from build123d import *

# Parameters (mm, degrees)
SCHIZZO1_W                   = 690
SCHIZZO1_H                   = 400
ESTRUSIONE_ESTRUSIONE1_DEPTH = 10
SCHIZZO2_W                   = 690
SCHIZZO2_H                   = 400
SCHIZZO2_W_2                 = 670
SCHIZZO2_H_2                 = 380
ESTRUSIONE_ESTRUSIONE2_DEPTH = 150


with BuildPart() as part:
    # Schizzo1 → Estrusione-Estrusione1 (new body)
    with BuildSketch(Plane.XY):
        Rectangle(SCHIZZO1_W, SCHIZZO1_H)
    extrude(amount=ESTRUSIONE_ESTRUSIONE1_DEPTH)

    # Schizzo2 → Estrusione-Estrusione2 (add)
    with BuildSketch(Plane.XY.offset(10)):
        Rectangle(SCHIZZO2_W, SCHIZZO2_H)
        Rectangle(SCHIZZO2_W_2, SCHIZZO2_H_2, mode=Mode.SUBTRACT)
    extrude(amount=ESTRUSIONE_ESTRUSIONE2_DEPTH)


solid = part.part
Can you work these out from the model? Positions are in its coordinate system, mm. A direction names the side the tool comes from. Coordinates: 2 decimals unless noted, no trailing zeros. Order: outer loops, then holes, each group sorted by start corner. A loop starts at its lowest first (then second) coordinate and runs counter-clockwise, first axis right, second up. Notation, with made-up numbers: (-40, 4) - (-29, 4) arc R26 cw to (-29, 21) - close; hole circle Ø2 at (6.5, 35). An arc over 180 degrees is marked (long way). Answer as a JSON object with one key per item and string values. Group by question number.
Q1. On a 3-axis mill with a long thin cutter (end or side, diameter ignored), from which of +Z, -Z, +X, -X, +Y, -Y can I reach the whole of each face in a straight line? I mean faces 1 (the face through (-345, -3, 79)), 2 (the face through (-5, 3, 10)). Say none if no direction works.
Q2. Imagine slicing it at A-A (z = 78). Please give me the cut outline in (x, y), and give its area (3 significant figures).
Q3. We'd pull the mould along X, two halves only. Please class faces 3 (the face through (345, -3, 79)), 4 (the face through (-5, -200, 79)), 5 (the face through (335, -3, 84)): +X half, -X half, draft (parallel to the pull), parting line (faces both ways), or undercut.
Q4. I need wall thicknesses on line 1 (X direction, y = 168.5, z = 129); line 2 (Y direction, x = -67.5, z = 119); line 3 (Z direction, x = 279.5, y = -92). Which ranges of each line are inside material? Lowest first, please. Write a range as from..to.
Q5. Imagine slicing it at B-B (y = -88.5). Please give me the cut outline in (x, z), and give its area (3 significant figures).
Q6. Imagine slicing it at C-C (x = -258). Please give me the cut outline in (y, z), and give its area (3 significant figures).
Q7. Will this pin go through, and if not, where does the flat tip stop? P1, Ø12, axis at x = -160, y = -2.5, coming from the -Z side.
Determined:
{
 "1": {"face 1": "+Z, -Z, -X, +Y, -Y", "face 2": "+Z"},
 "2": {"outline": "(-345, -200) - (345, -200) - (345, 200) - (-345, 200) - close; hole (-335, -190) - (335, -190) - (335, 190) - (-335, 190) - close", "area": "21,400 mm2"},
 "3": {"face 3": "+X half", "face 4": "draft", "face 5": "undercut"},
 "4": {"line 1": "x = -345..-335, 335..345", "line 2": "y = -200..-190, 190..200", "line 3": "z = 0..10"},
 "5": {"outline": "(-345, 0) - (345, 0) - (345, 160) - (335, 160) - (335, 10) - (-335, 10) - (-335, 160) - (-345, 160) - close", "area": "9,900 mm2"},
 "6": {"outline": "(-200, 0) - (200, 0) - (200, 160) - (190, 160) - (190, 10) - (-190, 10) - (-190, 160) - (-200, 160) - close", "area": "7,000 mm2"},
 "7": {"P1": "stops at z = 0"}
}
